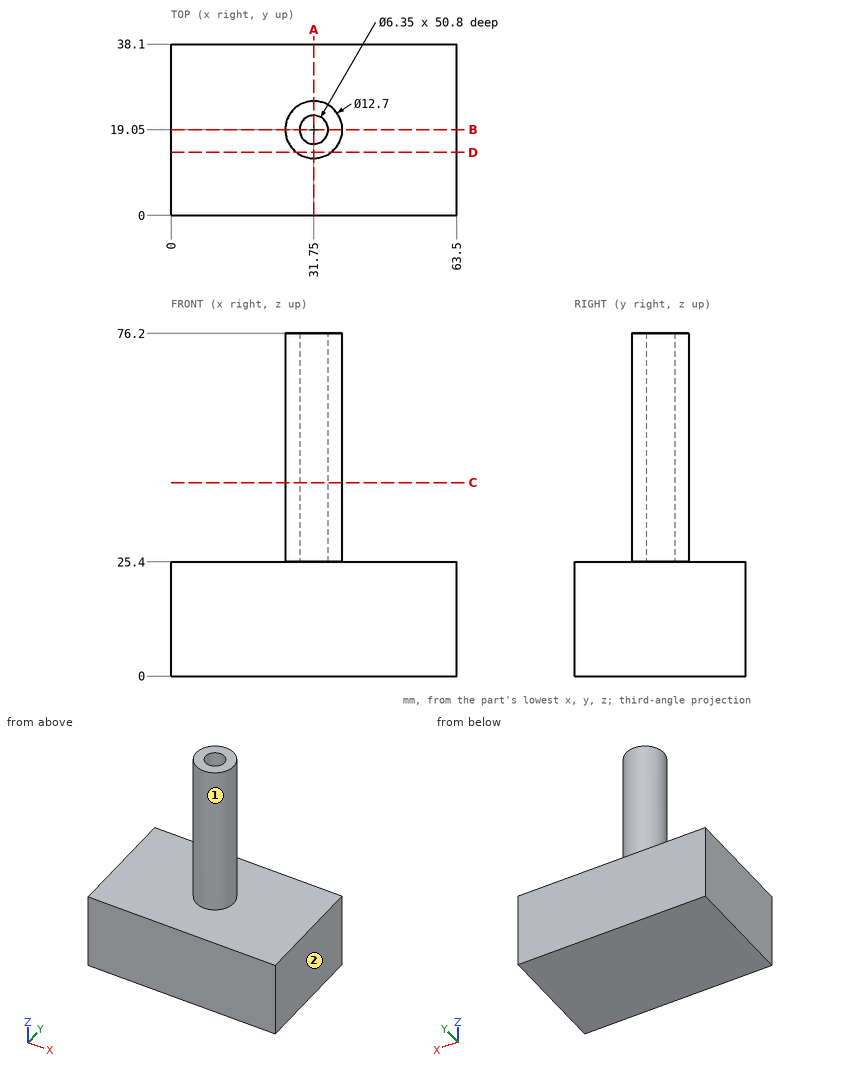
Source: three-view drawing plus pictorial views. Frame: mm from the lowest corner of the part. A direction names the side the tool comes from. Round coordinates to 2 decimals unless told otherwise and drop trailing zeros. Loops run counter-clockwise (first coordinate to the right, second up) from the corner with the lowest first, then second, coordinate; pieces in that order, holes last.
Q1. Section D-D on y = 14. Return loops of the section in (x, z).
Q2. Section A-A on x = 31.75. Return loops of the section in (y, z) (3 decimals).
Q3. Pin query (flat end, axial travel): P1, Ø6, axis at x = 47.5, y = 28.5, coming from the +Z side; P2, Ø10, axis at x = 31.75, y = 19.05, coming from the -Z side; P3, Ø8, axis at x = 31, z = 37.5, coming from the +Y side; P4, Ø5, axis at x = 26, z = 65, coming from the +Y side. Return the tip coordinate at first contact, or that it passes through.
Q4. Access query for the marked faces 1 and 2. Directions: +Z, -Z, +X, -X, +Y, -Y. A direction counts if a zero-diameter tool reaches every point of the face in a straight line with its end or side. Return the directions, or none.
Q5. Section B-B on y = 19.05. Return loops of the section in (x, z) (3 decimals), plus the area to 3 significant figures.
Q6. Material intervals for L1, parallel to X at y = 19, z = 53; L2, parallel to Y at x = 31.75, z = 47.5 (3 decimals); L3, parallel to Z at x = 38, y = 3, sorted ascending.
Q7. Section C-C on z = 43. Return loops of the section in (x, y) (3 decimals).
Evaluation:
1. outline: (0, 0) - (63.5, 0) - (63.5, 25.4) - (35.6, 25.4) - (35.6, 76.2) - (27.9, 76.2) - (27.9, 25.4) - (0, 25.4) - close
2. outline: (0, 0) - (38.1, 0) - (38.1, 25.4) - (25.4, 25.4) - (25.4, 76.2) - (22.225, 76.2) - (22.225, 25.4) - (15.875, 25.4) - (15.875, 76.2) - (12.7, 76.2) - (12.7, 25.4) - (0, 25.4) - close
3. P1: stops at z = 25.4
3. P2: stops at z = 0
3. P3: stops at y = 25.4
3. P4: stops at y = 24.51
4. face 1: +Z
4. face 2: +Z, -Z, +X, +Y, -Y
5. outline: (0, 0) - (63.5, 0) - (63.5, 25.4) - (38.1, 25.4) - (38.1, 76.2) - (34.925, 76.2) - (34.925, 25.4) - (28.575, 25.4) - (28.575, 76.2) - (25.4, 76.2) - (25.4, 25.4) - (0, 25.4) - close
5. area: 1,940 mm2
6. L1: x = 25.4 to 28.58, 34.92 to 38.1
6. L2: y = 12.7 to 15.875, 22.225 to 25.4
6. L3: z = 0 to 25.4
7. outline: circle Ø12.7 at (31.75, 19.05); hole circle Ø6.35 at (31.75, 19.05)
